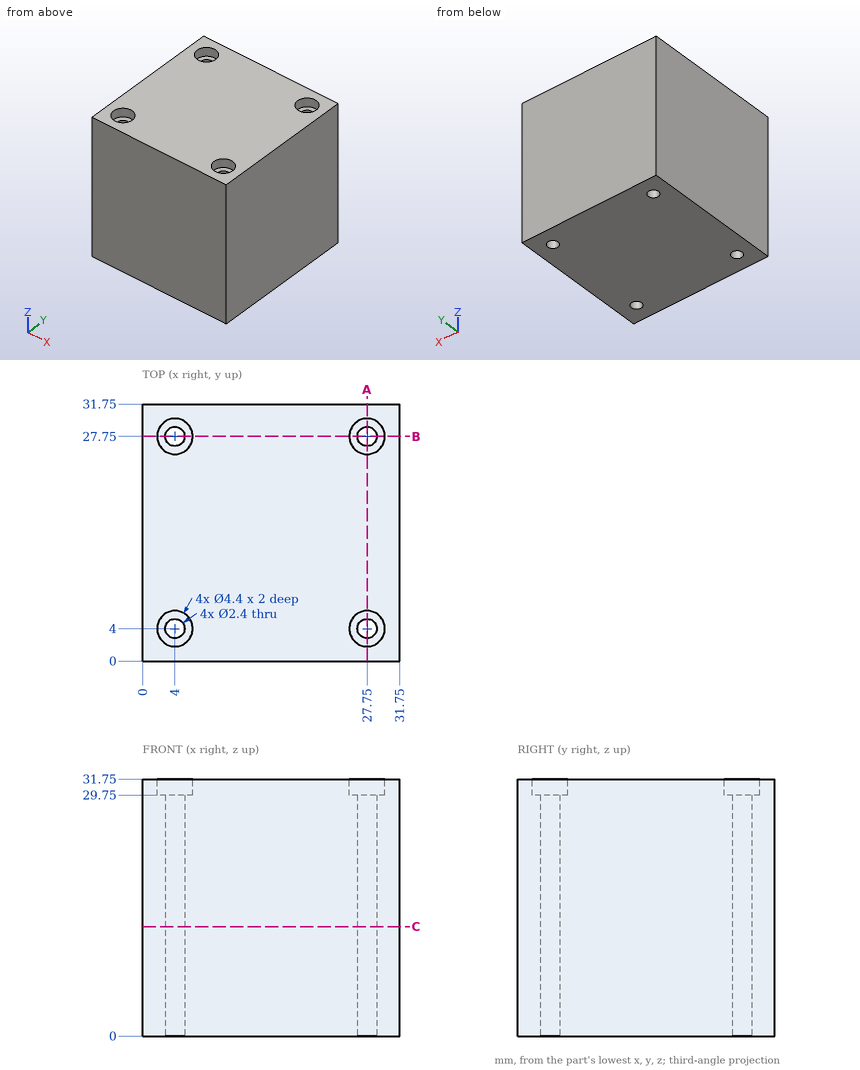
Geometry check sheet. Reference: drawing and pictorial views, mm from the part's lowest x, y, z. Give positions to 0.01 mm unless a question says otherwise; leave off trailing zeros. Order: outer loops, then holes, each group sorted by start corner. A loop starts at its lowest first (then second) coordinate and runs counter-clockwise, first axis right, second up. Notation, with made-up numbers: M -35,-7 L -18,-7 A28 ccw -18,11 Z; hole C 53.25,73.5 d5. An arc over 180 degrees is marked long. Answer in a Markdown table with one row per item. Add a question column.
Item 1: Section check C-C, the plane z = 13.5. Enter the section's corners in (x, y).
Item 2: Gauge pin test, flat ends, axial feed: pin 1 (1.4 mm diameter, centred on x = 27.75, y = 4, fed in from +Z); pin 2 (2.5 mm diameter, centred on x = 4, y = 27.75, fed in from +Z). Record the tip position at first contact, or that the pin passes through.
Item 3: Section check A-A, the plane x = 27.75. Enter the section's corners in (y, z), and give its area (3 significant figures).
Item 4: Scan lines: probe 1 along Y at (x, z) = (4, 31); probe 2 along Y at (x, z) = (28.5, 14); probe 3 along X at (y, z) = (27.5, 2.5). Record each from-to range of solid material in increasing order. Write a range as from..to.
Filled sheet:
| question | item | result |
|---|---|---|
| 1 | outline | M 0,0 L 31.75,0 L 31.75,31.75 L 0,31.75 Z; hole C 4,4 d2.4; hole C 4,27.75 d2.4; hole C 27.75,4 d2.4; hole C 27.75,27.75 d2.4 |
| 2 | pin 1 | passes through |
| 2 | pin 2 | stops at z = 29.75 |
| 3 | outline | M 0,0 L 2.8,0 L 2.8,29.75 L 1.8,29.75 L 1.8,31.75 L 0,31.75 Z; M 5.2,0 L 26.55,0 L 26.55,29.75 L 25.55,29.75 L 25.55,31.75 L 6.2,31.75 L 6.2,29.75 L 5.2,29.75 Z; M 28.95,0 L 31.75,0 L 31.75,31.75 L 29.95,31.75 L 29.95,29.75 L 28.95,29.75 Z |
| 3 | area | 848 mm^2 |
| 4 | probe 1 | y = 0..1.8, 6.2..25.55, 29.95..31.75 |
| 4 | probe 2 | y = 0..3.06, 4.94..26.81, 28.69..31.75 |
| 4 | probe 3 | x = 0..2.83, 5.17..26.58, 28.92..31.75 |
